Autodesk Inventor part; units mm, degrees
ref_plane "YZ Plane" through (0, 0, 0) normal (1, 0, 0) x (0, 1, 0)
ref_plane "XZ Plane" through (0, 0, 0) normal (0, 1, 0) x (-1, 0, 0)
ref_plane "XY Plane" through (0, 0, 0) normal (0, 0, 1) x (1, 0, 0)
sketch "Sketch1" plane through (0, 0, 0) normal (0, 0, 1) x (1, 0, 0)
  circle A0 centre (0, 0) radius 73.025
  dimension "d7" = 146.05
extrude "Plate1" add sketch "Sketch1" along normal blind 4.7625
sketch "Sketch2" plane through (0, 0, 4.7625) normal (0, 0, 1) x (1, 0, 0)
  circle A0 centre (-11.2011, 7.8489) radius 3.9688
  circle A1 centre (-7.8489, -11.2011) radius 3.9688
  circle A2 centre (11.2011, -7.8489) radius 3.9688
  circle A3 centre (7.8489, 11.2011) radius 3.9688
  point P0 (0, 0)
  dimension "d8" = 7.9375
  dimension "d11" = 360
  dimension "d20" = 19.05
hole "Hole1" at (-11.2011, 7.8489, 4.7625) at (7.8489, 11.2011, 4.7625) at (-7.8489, -11.2011, 4.7625) at (11.2011, -7.8489, 4.7625) direction (0, 0, -1) diameter 7.9375 end through all
sketch "Sketch3" plane through (0, 0, 4.7625) normal (0, 0, 1) x (1, 0, 0)
  circle A0 centre (-34.3723, 46.8025) radius 6.498 construction
  circle A1 centre (-55.1334, -18.2273) radius 6.498 construction
  circle A2 centre (0.298, -58.0676) radius 6.498 construction
  circle A3 centre (55.3176, -17.6604) radius 6.498 construction
  circle A4 centre (33.8902, 47.1528) radius 6.498 construction
  point P0 (0, 0)
  dimension "d21" = 12.9959
  dimension "d24" = 360
  dimension "d33" = 68.2625
hole "Hole2" at (33.8902, 47.1528, 4.7625) at (55.3176, -17.6604, 4.7625) at (0.298, -58.0676, 4.7625) at (-55.1334, -18.2273, 4.7625) at (-34.3723, 46.8025, 4.7625) direction (0, 0, -1) diameter 14.2875 end through all
equation "\"d18\" = Thickness"
equation "\"d31\" = Thickness"
equation "\"BendRadius\" = Thickness"
equation "\"BendReliefWidth\" = Thickness"
equation "\"BendReliefDepth\" = 0.5 * Thickness"
equation "\"CornerReliefSize\" = 4 * Thickness"
equation "\"MinimumRemnant\" = 2 * Thickness"
equation "\"TransitionRadius\" = BendRadius"
equation "\"JacobiRadiusSize\" = BendRadius"
equation "\"GapSize\" = Thickness"
equation "\"d0\" = BendRadius"
properties part number "WheelHub" material "Steel, Mild"
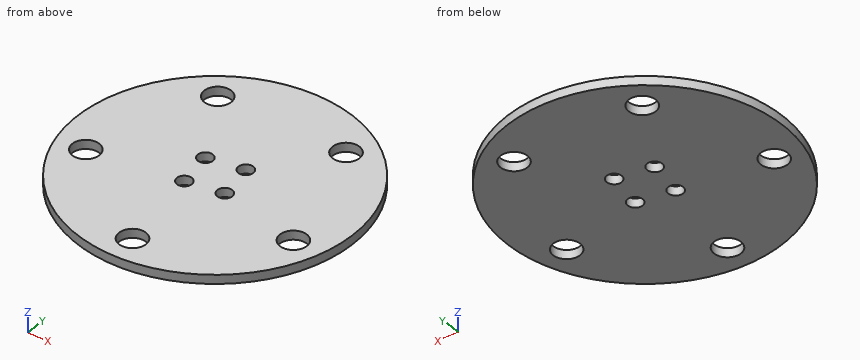
Input: part model. Units: mm. Frame: model coordinates. Give positions to 0.01 mm unless a question says otherwise; leave off trailing zeros. Loops run counter-clockwise (first coordinate to the right, second up) from the corner with the lowest first, then second, coordinate; pieces in that order, holes last. Notation, with made-up numbers: (74.25, 63.5) - (127.25, 63.5) arc R15 ccw to (127.25, 79.5) - close; hole circle Ø2 at (-10.75, 0.25). An arc over 180 degrees is marked (long way). Use CSV: the item, a comma, the result in double quotes. Start each with the question number.
Item 1: Section A-A on z = 1.7. State how many separate pieces and enclosed holes the cut face has, then the cut area to 3 significant figures.
Item 2: Contact query for flat-ended pins moving along their axis: P1, Ø1, axis at y = -23.5, z = 3.5, coming from the -X side; P2, Ø1.5, axis at y = 6, z = 2.5, coming from the -X side; P3, Ø1, axis at y = 2, z = 1, coming from the +X side. Output: stop coordinate, or through.
Item 3: Section B-B on x = -24.5. Return loops of the section in (y, z), then the cut area to 3 significant figures.
Item 4: Line query: line 1 (X direction, y = -14, z = 2); line 2 (X direction, y = -20, z = 1.4); line 3 (X direction, y = -19.5, z = 1.8). Output: solid intervals per line, ascending.
Item 5: Section C-C on y = 64.5. Return loops of the section in (x, z), then the cut area to 3 significant figures.
Ans:
1,separate pieces,"1"
1,enclosed holes,"9"
1,area,"15,800 mm2"
2,P1,"stops at x = -69.31"
2,P2,"stops at x = -72.84"
2,P3,"stops at x = 73.01"
3,outline,"(-68.79, 0) - (68.79, 0) - (68.79, 4.76) - (-68.79, 4.76) - close"
3,area,"655 mm2"
4,line 1,"x = -71.67 to -60.89, -49.37 to -10.66, -5.04 to 49.18, 61.45 to 71.67"
4,line 2,"x = -70.23 to -62.05, -48.21 to 48.57, 62.07 to 70.23"
4,line 3,"x = -70.37 to -62.16, -48.1 to 48.41, 62.22 to 70.37"
5,outline,"(-34.24, 0) - (34.24, 0) - (34.24, 4.76) - (-34.24, 4.76) - close"
5,area,"326 mm2"
